Verification items for the finished model (mm, model axes). Coordinates: 2 decimals unless noted, no trailing zeros. Order: outer loops, then holes, each group sorted by start corner. A loop starts at its lowest first (then second) coordinate and runs counter-clockwise, first axis right, second up. Notation, with made-up numbers: (33.25, -14) - (55.25, -14) arc R16 ccw to (55.25, 7) - close; hole circle Ø3 at (-1.5, -33). An arc over 180 degrees is marked (long way). Answer as CSV lines item,"result". Start each with the question number.
1. Section check C-C (y = 0). Record the cut outline in (x, z), and give its area (3 significant figures).
2. Go/stop test with flat-tipped pins: pin 1 (9 mm diameter, centred on x = 0, y = 0, fed in from -Z); pin 2 (1.5 mm diameter, centred on y = -44, z = 1.5, fed in from +X); pin 3 (1.5 mm diameter, centred on y = 45, z = 2, fed in from -X). Record where each tip stops, or that it passes through.
3. Section check A-A (y = -44.75). Record the cut outline in (x, z), and give its area (3 significant figures).
4. Material ranges on L1, parallel to Y at x = 0, z = 0.75; L2, parallel to Y at x = 44.75, z = 1.4; L3, parallel to X at y = -44, z = 2.15, recorded low to high. Write a range as [from, to].
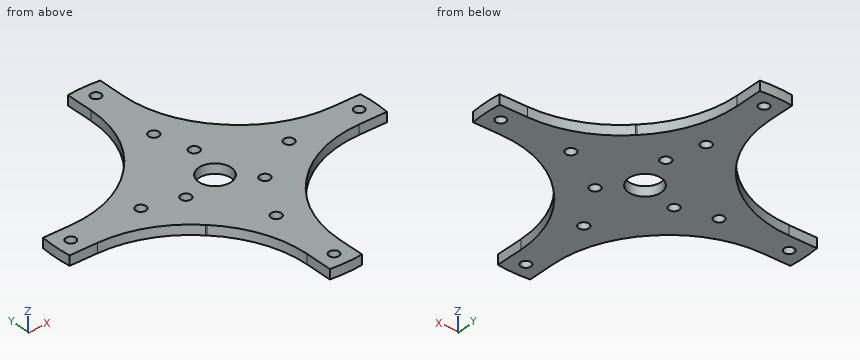
from build123d import *

# Parameters (mm, degrees)
SKETCH_1_R          = 1.55
SKETCH_1_R_2        = 5
SKETCH_1_R_3        = 1.6
EXTRUDE_1_DEPTH     = 3
FILLET_1_R          = 35
SKETCH_2_R          = 1.6
CUT_EXTRUDE_1_DEPTH = 14


with BuildPart() as part:
    # 草图1 → 凸台-拉伸1 (new body)
    with BuildSketch(Plane.XY):
        with BuildLine():
            Line((49.246827309, 5), (21.424285286, 5))
            ThreePointArc((21.424285286, 5), (15.556349186, 15.556349186), (5, 21.424285286))
            Line((5, 21.424285286), (5, 49.246827309))
            ThreePointArc((5, 49.246827309), (0, 49.5), (-5, 49.246827309))
            Line((-5, 49.246827309), (-5, 21.424285286))
            ThreePointArc((-5, 21.424285286), (-15.556349186, 15.556349186), (-21.424285286, 5))
            Line((-21.424285286, 5), (-49.246827309, 5))
            ThreePointArc((-49.246827309, 5), (-49.5, 0), (-49.246827309, -5))
            Line((-49.246827309, -5), (-21.424285286, -5))
            ThreePointArc((-21.424285286, -5), (-15.556349186, -15.556349186), (-5, -21.424285286))
            Line((-5, -21.424285286), (-5, -49.246827309))
            ThreePointArc((-5, -49.246827309), (0, -49.5), (5, -49.246827309))
            Line((5, -49.246827309), (5, -21.424285286))
            ThreePointArc((5, -21.424285286), (15.556349186, -15.556349186), (21.424285286, -5))
            Line((21.424285286, -5), (49.246827309, -5))
            ThreePointArc((49.246827309, -5), (49.5, 0), (49.246827309, 5))
        make_face()
        with Locations((-44.75, 0)):
            Circle(SKETCH_1_R, mode=Mode.SUBTRACT)
        Circle(SKETCH_1_R_2, mode=Mode.SUBTRACT)
        with Locations((0, 44.75)):
            Circle(SKETCH_1_R, mode=Mode.SUBTRACT)
        with Locations((44.75, 0)):
            Circle(SKETCH_1_R, mode=Mode.SUBTRACT)
        with Locations((0, -44.75)):
            Circle(SKETCH_1_R, mode=Mode.SUBTRACT)
        with Locations((3.105828541, 11.591109915)):
            Circle(SKETCH_1_R_3, mode=Mode.SUBTRACT)
        with Locations((8.485281374, -8.485281374)):
            Circle(SKETCH_1_R_3, mode=Mode.SUBTRACT)
        with Locations((-11.591109915, -3.105828541)):
            Circle(SKETCH_1_R_3, mode=Mode.SUBTRACT)
    extrude(amount=EXTRUDE_1_DEPTH)

    # 圆角1
    fillet_1_edges = [part.edges().sort_by_distance(p)[0] for p in [
        (5, 21.424285286, 1.5),
        (21.424285286, 5, 1.5),
        (21.424285286, -5, 1.5),
        (5, -21.424285286, 1.5),
        (-5, -21.424285286, 1.5),
        (-21.424285286, -5, 1.5),
        (-21.424285286, 5, 1.5),
        (-5, 21.424285286, 1.5),
    ]]
    fillet(fillet_1_edges, radius=FILLET_1_R)

    # 草图2 → 切除-拉伸1 (cut)
    with BuildSketch(Plane.XY.offset(3)):
        with Locations((-23, 0)):
            Circle(SKETCH_2_R)
        with Locations((0, 23)):
            Circle(SKETCH_2_R)
        with Locations((23, 0)):
            Circle(SKETCH_2_R)
        with Locations((0, -23)):
            Circle(SKETCH_2_R)
    extrude(amount=-CUT_EXTRUDE_1_DEPTH, mode=Mode.SUBTRACT)


solid = part.part
Evaluation:
1,outline,"(-49.5, 0) - (-46.3, 0) - (-46.3, 3) - (-49.5, 3) - close; (-43.2, 0) - (-24.6, 0) - (-24.6, 3) - (-43.2, 3) - close; (-21.4, 0) - (-5, 0) - (-5, 3) - (-21.4, 3) - close; (5, 0) - (21.4, 0) - (21.4, 3) - (5, 3) - close; (24.6, 0) - (43.2, 0) - (43.2, 3) - (24.6, 3) - close; (46.3, 0) - (49.5, 0) - (49.5, 3) - (46.3, 3) - close"
1,area,"229 mm²"
2,pin 1,"passes through"
2,pin 2,"stops at x = 5"
2,pin 3,"stops at x = -5"
3,outline,"(-5, 0) - (-1.55, 0) - (-1.55, 3) - (-5, 3) - close; (1.55, 0) - (5, 0) - (5, 3) - (1.55, 3) - close"
3,area,"20.7 mm²"
4,L1,"y = [-49.5, -46.3], [-43.2, -24.6], [-21.4, -5], [5, 21.4], [24.6, 43.2], [46.3, 49.5]"
4,L2,"y = [-5, -1.55], [1.55, 5]"
4,L3,"x = [-5, -1.36], [1.36, 5]"
